The model under review builds one solid part; all positions refer to its coordinate system, in mm. Face numbers are marked on the shaded views. A direction names the side the tool comes from. Round coordinates to 2 decimals unless told otherwise and drop trailing zeros. Order: outer loops, then holes, each group sorted by start corner. A loop starts at its lowest first (then second) coordinate and runs counter-clockwise, first axis right, second up. Notation, with made-up numbers: (8, 86) -> (67, 86) arc R23 ccw to (67, 114) -> close; hole circle Ø1 at (40, 66). An arc over 180 degrees is marked (long way). Put each result on its own line as item: value. Start each with the question number.
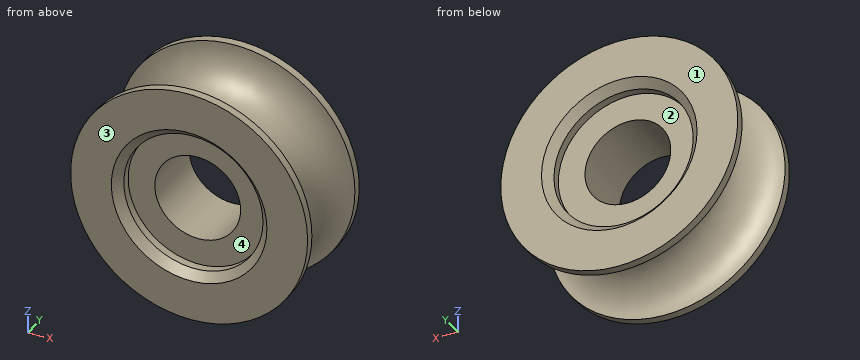
from build123d import *

# Parameters (mm, degrees)
F0_R     = 14.5
F1_DEPTH = 12
F2_W     = 5.25
F2_H     = 8
F2_R     = 5
F4_SIZE  = 1


with BuildPart() as f1:
    # F0 (on Front) → F1 (new body)
    with BuildSketch(Plane.XZ):
        Circle(F0_R)
    extrude(amount=F1_DEPTH)

    # F2 (on Top) → F3 (revolve, cut)
    with BuildSketch(Plane.XY):
        with Locations((2.625, -6)):
            Rectangle(F2_W, F2_H)
        Polygon((5.25, -10), (0, -10), (0, -12.965777), (8.519073, -12.965777), (8.519073, -10), align=None)
        Polygon((0, 0), (0, -2), (5.25, -2), (8.519073, -2), (8.519073, 0), align=None)
        with Locations((14.5, -6)):
            Circle(F2_R)
    revolve(axis=Axis((0, -8.281275, 0), (0, -1, 0)), mode=Mode.SUBTRACT)

    # F4
    f4_edges = [f1.edges().sort_by_distance(p)[0] for p in [
        (-8.519073, 0, 0),
        (-8.519073, -12, 0),
    ]]
    chamfer(f4_edges, length=F4_SIZE)


solid = f1.part
Q1. Clearance check with flat-ended pins moving along their axes: pin 1 Ø4 at (x, y) = (-8.5, -4) entering from -Z; pin 2 Ø13.5 at (x, z) = (0, 0) entering from -Y; pin 3 Ø8 at (x, z) = (-5.5, -6.5) entering from +Y; pin 4 Ø10 at (x, z) = (0, 0) entering from +Y. State where each tip first meets the part, or that it passes through.
Q2. Take a section at B-B on x = 0. Give the boundary of the cut face in (y, z).
Q3. Take a section at C-C on y = -2.5. Give the boundary of the cut face in (x, z), and give its area (3 significant figures).
Q4. Take a section at A-A on z = 0. Give the boundary of the cut face in (x, y), and give its area (3 significant figures).
Q5. Wall thickness on probe 1 along Y at (x, z) = (-2.75, -5.5); probe 2 along Z at (x, y) = (1.5, -6.5); probe 3 along Z at (x, y) = (-2.75, -4.5): over which ranges is each line inside the solid? List them lowest first. Write a range as [from, to].
Q6. For the marked faces 1 and 2, list the 3-axis set-ups (+Z, -Z, +X, -X, +Y, -Y) from which the entire face can be reached by the end or side of a thin tool; tool diameter is ignored.
Q7. Draft analysis for pull direction X (two halves, no side actions). For the marked faces 3 and 4, state which applies: +X half, -X half, draft (parallel to the pull), parting line (faces both ways), or undercut.
Q8. Take a section at D-D on y = -7. Give the boundary of the cut face in (x, z).
Calculated:
1. pin 1: stops at z = -8.28
1. pin 2: stops at y = -10
1. pin 3: stops at y = 0
1. pin 4: passes through
2. outline: (-12, -14.5) -> (-11, -14.5) arc R5 cw to (-1, -14.5) -> (0, -14.5) -> (0, -9.52) -> (-1, -8.52) -> (-2, -8.52) -> (-2, -5.25) -> (-10, -5.25) -> (-10, -8.52) -> (-11, -8.52) -> (-12, -9.52) -> close; (-12, 9.52) -> (-11, 8.52) -> (-10, 8.52) -> (-10, 5.25) -> (-2, 5.25) -> (-2, 8.52) -> (-1, 8.52) -> (0, 9.52) -> (0, 14.5) -> (-1, 14.5) arc R5 cw to (-11, 14.5) -> (-12, 14.5) -> close
3. outline: circle Ø21.86 at (0, 0); hole circle Ø10.5 at (0, 0)
3. area: 289 mm²
4. outline: (-14.5, -12) -> (-9.52, -12) -> (-8.52, -11) -> (-8.52, -10) -> (-5.25, -10) -> (-5.25, -2) -> (-8.52, -2) -> (-8.52, -1) -> (-9.52, 0) -> (-14.5, 0) -> (-14.5, -1) arc R5 cw to (-14.5, -11) -> close; (5.25, -10) -> (8.52, -10) -> (8.52, -11) -> (9.52, -12) -> (14.5, -12) -> (14.5, -11) arc R5 cw to (14.5, -1) -> (14.5, 0) -> (9.52, 0) -> (8.52, -1) -> (8.52, -2) -> (5.25, -2) -> close
4. area: 115 mm²
5. probe 1: y = [-10, -2]
5. probe 2: z = [-9.41, -5.03], [5.03, 9.41]
5. probe 3: z = [-9.33, -4.47], [4.47, 9.33]
6. face 1: +Z, -Z, +X, -X, +Y
6. face 2: +Y
7. face 3: draft
7. face 4: undercut
8. outline: circle Ø19.2 at (0, 0); hole circle Ø10.5 at (0, 0)
